Autodesk Inventor part; units mm, degrees
ref_plane "YZ Plane" through (0, 0, 0) normal (1, 0, 0) x (0, 1, 0)
ref_plane "XZ Plane" through (0, 0, 0) normal (0, 1, 0) x (-1, 0, 0)
ref_plane "XY Plane" through (0, 0, 0) normal (0, 0, 1) x (1, 0, 0)
sketch "Esboço1" plane through (0, 0, 0) normal (0, 1, 0) x (-1, 0, 0)
  line L0 (-40, 40) -> (40, 40)
  line L1 (40, 40) -> (40, -40)
  line L2 (40, -40) -> (-40, -40)
  line L3 (-40, -40) -> (-40, 40)
  line L4 (-40, 40) -> (40, -40) construction
  line L5 (40, 40) -> (-40, -40) construction
  point P0 (0, 0)
  dimension "d0" = 80
  dimension "d1" = 80
extrude "Extrusão1" add sketch "Esboço1" along normal blind 2.5
sketch "Esboço2" plane through (0, 2.5, 0) normal (0, 1, 0) x (1, 0, 0)
  circle A0 centre (33, -28) radius 1.5875
  line L0 (-40, -40) -> (40, -40)
  line L1 (40, -40) -> (40, 40)
  circle A1 centre (33, -0.06) radius 1.5875
  circle A2 centre (33, -28) radius 4.5
  circle A3 centre (33, -0.06) radius 4.5
  dimension "d4" = 3.175
  dimension "d5" = 12
  dimension "d6" = 7
  dimension "d7" = 3.175
  dimension "d8" = 27.94
  dimension "d9" = 9
  dimension "d10" = 9
extrude "Extrusão2" add sketch "Esboço2" along normal blind 3
sketch "Esboço3" plane through (0, 2.5, 0) normal (0, 1, 0) x (1, 0, 0)
  line L0 (-6.9727, -23.0834) -> (-13.0273, -23.0834)
  line L1 (-13.0273, -23.0834) -> (-13.0273, 3.9103)
  line L2 (-13.0273, 3.9103) -> (-6.9727, 3.9103)
  line L3 (-6.9727, 3.9103) -> (-6.9727, -23.0834)
  line L4 (-6.9727, -23.0834) -> (-13.0273, 3.9103) construction
  line L5 (-13.0273, -23.0834) -> (-6.9727, 3.9103) construction
  line L6 (40, -40) -> (40, 40)
  point P0 (0, 0)
  point P1 (-10, -9.5866)
  dimension "d13" = 50
extrude "Extrusão3" add sketch "Esboço3" along normal blind 3
sketch "Esboço4" plane through (0, 2.5, 0) normal (0, 1, 0) x (1, 0, 0)
  line L0 (13, 36) -> (-15, 36)
  line L1 (-15, 36) -> (-15, 22)
  line L2 (-15, 22) -> (13, 22)
  line L3 (13, 22) -> (13, 36)
  line L4 (35.54, 17.72) -> (-33.04, 17.72)
  line L5 (-33.04, 17.72) -> (-33.04, -35.62)
  line L6 (-33.04, -35.62) -> (35.54, -35.62)
  line L7 (35.54, -35.62) -> (35.54, 17.72)
  circle A0 centre (33, -28) radius 1.5875
  line L8 (15, 38) -> (-17, 38)
  line L9 (-17, 38) -> (-17, 20)
  line L10 (-17, 20) -> (15, 20)
  line L11 (15, 20) -> (15, 38)
  line L12 (40, 40) -> (-40, 40)
  line L13 (40, -40) -> (40, 40)
  point P0 (0, 0)
  dimension "d16" = 28
  dimension "d17" = 14
  dimension "d18" = 68.58
  dimension "d19" = 53.34
  dimension "d20" = 7.62
  dimension "d21" = 2.54
  dimension "d22" = 4
  dimension "d23" = 27
  dimension "d24" = 2
  dimension "d25" = 2
  dimension "d26" = 2
  dimension "d27" = 2
extrude "Extrusão4" add sketch "Esboço4" along normal blind 6 contours L11 L10 L9 L8
sketch "Esboço5" plane through (-17, 2.5, -20) normal (0, 0, 1) x (1, 0, 0)
  line L0 (0, 6) -> (32, 6)
  line L1 (3.1604, 6) -> (8.0765, 6)
  line L2 (8.0765, 6) -> (8.0765, 3)
  line L3 (8.0765, 3) -> (3.1604, 3)
  line L4 (3.1604, 3) -> (3.1604, 6)
  point P0 (17, -2.5)
  dimension "d32" = 3
extrude "Extrusão5" cut sketch "Esboço5" against normal blind 6
sketch "Esboço6" plane through (0, 2.5, 0) normal (0, 1, 0) x (1, 0, 0)
  line L0 (15, 20) -> (-17, 20)
  line L1 (-17, 20) -> (-27, 20)
  line L2 (-27, 20) -> (-27, 38)
  line L3 (-27, 38) -> (-17, 38)
  line L4 (-17, 38) -> (-17, 20)
  point P0 (0, 0)
  dimension "d33" = 10
extrude "Extrusão6" add sketch "Esboço6" along normal blind 6
fillet "Arredondamento1" radius 9 2 edges at (-27, 5.5, -20) (-27, 5.5, -38)
sketch "Esboço7" plane through (0, 8.5, 0) normal (0, 1, 0) x (1, 0, 0)
  circle A0 centre (-19.962, 29) radius 1.5
  point P0 (0, 0)
  dimension "d37" = 3
extrude "Extrusão7" cut sketch "Esboço7" against normal blind 6
sketch "Esboço8" plane through (0, 2.5, 0) normal (0, 1, 0) x (1, 0, 0)
  line L0 (-42.5, -42.5) -> (42.5, -42.5)
  line L1 (42.5, -42.5) -> (42.5, 42.5)
  line L2 (42.5, 42.5) -> (-42.5, 42.5)
  line L3 (-42.5, 42.5) -> (-42.5, -42.5)
  line L4 (40, 40) -> (-40, 40)
  line L5 (-40, 40) -> (-40, -40)
  line L6 (-40, -40) -> (40, -40)
  line L7 (40, -40) -> (40, 40)
  point P0 (0, 0)
  dimension "d40" = 2.5
  dimension "d41" = 2.5
  dimension "d42" = 2.5
  dimension "d43" = 2.5
extrude "Extrusão8" add sketch "Esboço8" along normal blind 25 and the other way blind 2.5
fillet "Arredondamento2" radius 2 4 edges at (-42.5, 13.75, 42.5) (-42.5, 13.75, -42.5) (42.5, 13.75, 42.5) (42.5, 13.75, -42.5)
sketch "Esboço10" plane through (-42.5, 0, -40.5) normal (-1, 0, 0) x (0, 0, 1)
  line L0 (76.52, 0) -> (23.18, 0)
  line L1 (81, 27.5) -> (81, 0)
  line L2 (0.5, 2.5) -> (80.5, 2.5)
  line L3 (32.58, 2.5) -> (47.58, 2.5)
  line L4 (47.58, 2.5) -> (47.58, 14.5)
  line L5 (47.58, 14.5) -> (32.58, 14.5)
  line L6 (32.58, 14.5) -> (32.58, 2.5)
  point P0 (40.5, 0)
  dimension "d51" = 15
  dimension "d52" = 12
extrude "Extrusão9" cut sketch "Esboço10" against normal blind 3
fillet "Arredondamento3" radius 2 2 edges at (-41.25, 14.5, 7.08) (-41.25, 14.5, -7.92)
sketch "Esboço11" plane through (0, 27.5, 0) normal (0, 1, 0) x (1, 0, 0)
  line L0 (40, -40) -> (40, 40)
  line L1 (40, 40) -> (34, 40)
  line L2 (34, 40) -> (34, 34)
  line L3 (34, 34) -> (40, 34)
  line L4 (40, 34) -> (40, 40)
  line L5 (-40, -7.08) -> (-40, -40)
  line L6 (-40, -40) -> (-34, -40)
  line L7 (-34, -40) -> (-34, -34)
  line L8 (-34, -34) -> (-40, -34)
  line L9 (-40, -34) -> (-40, -40)
  point P0 (0, 0)
  dimension "d57" = 6
  dimension "d58" = 6
  dimension "d59" = 6
  dimension "d60" = 6
extrude "Extrusão10" add sketch "Esboço11" against normal blind 25
fillet "Arredondamento4" radius 2 2 edges at (-34, 15, 34) (34, 15, -34)
sketch "Esboço12" plane through (0, 27.5, 0) normal (0, 1, 0) x (1, 0, 0)
  circle A0 centre (-38.25, -38.25) radius 1.5
  circle A1 centre (38.25, 38.25) radius 1.5
  line L0 (40.5, 42.5) -> (-40.5, 42.5)
  line L1 (42.5, -40.5) -> (42.5, 40.5)
  line L2 (-40.5, -42.5) -> (40.5, -42.5)
  line L3 (-42.5, 40.5) -> (-42.5, -40.5)
  point P0 (0, 0)
  dimension "d64" = 3
  dimension "d65" = 3
  dimension "d66" = 4.25
  dimension "d67" = 4.25
  dimension "d68" = 4.25
  dimension "d69" = 4.25
extrude "Extrusão11" cut sketch "Esboço12" against normal blind 10
sketch "Esboço13" plane through (40.5, 0, -42.5) normal (0, 0, -1) x (-1, 0, 0)
  circle A0 centre (73.7947, 8.7851) radius 2.5
  point P0 (40.5, 0)
  dimension "d72" = 5
extrude "Extrusão12" cut sketch "Esboço13" against normal blind 10
properties part number "caixa box"
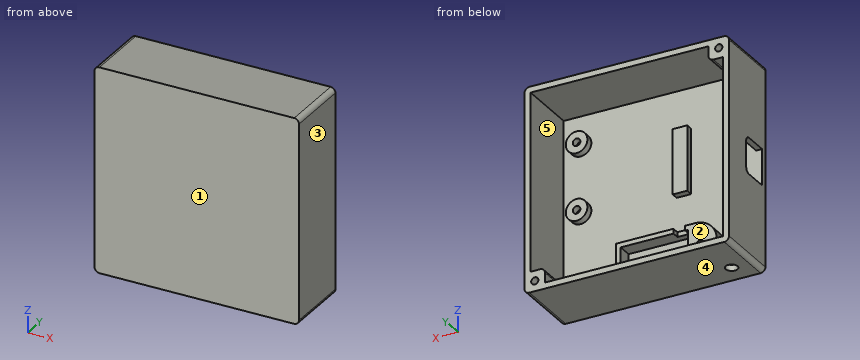
The model under review builds one solid part; all positions refer to its coordinate system, in mm. Face numbers are marked on the shaded views. A direction names the side the tool comes from. Coordinates: 2 decimals unless noted, no trailing zeros. Write each loop counter-clockwise with the first axis right and the second up, starting at its lowest first coordinate (ties: lowest second). Pieces come first, ordered by that corner, then holes. Notation, with made-up numbers: (22, 42.5) - (76, 42.5) arc R7 cw to (76, 53.5) - close; hole circle Ø1 at (66, -39.5). An arc over 180 degrees is marked (long way). Answer in a Markdown table with one row per item. Add a question column.
Q1. For the marked faces 1 and 2, list the 3-axis set-ups (+Z, -Z, +X, -X, +Y, -Y) from which the entire face can be reached by the end or side of a thin tool; tool diameter is ignored.
Q2. To check wall thickness, follow line 1 along X through (y, z) = (25, 38.25); line 2 along Z through (x, y) = (-38.25, 21); line 3 along X through (y, z) = (4.65, 0.06). State the ranges of each line that lie inside material, in increasing order. Write a range as from..to.
Q3. Clearance check with flat-ended pins moving along their axes: pin 1 (2 mm diameter, centred on x = -12, z = -21, fed in from +Y); pin 2 (8 mm diameter, centred on x = 33, z = -19.5, fed in from -Y); pin 3 (1 mm diameter, centred on x = -21.5, z = -22, fed in from +Y); pin 4 (0.8 mm diameter, centred on x = -41.5, y = 8.5, fed in from -Z). State where each tip first meets the part, or that it passes through.
Q4. Consider section B-B on y = 24.75. Give the boundary of the cut face in (x, z).
Q5. Draft analysis for pull direction X (two halves, no side actions). For the marked faces 3, 4 and 5, state which applies: +X half, -X half, draft (parallel to the pull), parting line (faces both ways), or undercut.
Q6. Consider section C-C on x = 4. Give the boundary of the cut face in (y, z).
Q7. Consider section A-A on z = 0.06. Give the boundary of the cut face in (x, y), then the cut area to 3 significant figures.
Q8. Consider section D-D on z = -10.5. Give the boundary of the cut face in (x, y), then the cut area to 4 significant figures.
Answers below:
| question | item | result |
|---|---|---|
| 1 | face 1 | +Z, -Z, +X, -X, -Y |
| 1 | face 2 | +Y |
| 2 | line 1 | -42.5..-39.75, -36.75..-34, 40..42.5 |
| 2 | line 2 | -42.5..-40, 34..36.75, 39.75..42.5 |
| 2 | line 3 | -13.03..-6.97, 28.5..31.41, 34.59..37.5, 40..42.5 |
| 3 | pin 1 | y = 5.5 |
| 3 | pin 2 | y = 0 |
| 3 | pin 3 | y = 8.5 |
| 3 | pin 4 | z = -42.41 |
| 4 | outline | (-42.5, -40.5) arc R2 ccw to (-40.5, -42.5) - (40.5, -42.5) arc R2 ccw to (42.5, -40.5) - (42.5, 40.5) arc R2 ccw to (40.5, 42.5) - (-40.5, 42.5) arc R2 ccw to (-42.5, 40.5) - close; hole (-40, -40) - (34, -40) - (34, -36) arc R2 cw to (36, -34) - (40, -34) - (40, 40) - (-34, 40) - (-34, 36) arc R2 cw to (-36, 34) - (-40, 34) - close; hole circle Ø3 at (-38.25, 38.25); hole circle Ø3 at (38.25, -38.25) |
| 5 | face 3 | +X half |
| 5 | face 4 | draft |
| 5 | face 5 | undercut |
| 6 | outline | (0, -42.5) - (27.5, -42.5) - (27.5, -40) - (2.5, -40) - (2.5, -38) - (8.5, -38) - (8.5, -36) - (2.5, -36) - (2.5, -22) - (8.5, -22) - (8.5, -20) - (2.5, -20) - (2.5, 40) - (27.5, 40) - (27.5, 42.5) - (0, 42.5) - close |
| 7 | outline | (-42.5, 0) - (42.5, 0) - (42.5, 27.5) - (40, 27.5) - (40, 2.5) - (37.5, 2.5) - (37.5, 5.5) - (34.59, 5.5) - (34.59, 2.5) - (31.41, 2.5) - (31.41, 5.5) - (28.5, 5.5) - (28.5, 2.5) - (-6.97, 2.5) - (-6.97, 5.5) - (-13.03, 5.5) - (-13.03, 2.5) - (-42.5, 2.5) - close; (-42.5, 14.5) - (-40, 14.5) - (-40, 27.5) - (-42.5, 27.5) - close |
| 7 | area | 343 mm² |
| 8 | outline | (-42.5, 0) - (42.5, 0) - (42.5, 27.5) - (40, 27.5) - (40, 2.5) - (-40, 2.5) - (-40, 27.5) - (-42.5, 27.5) - close |
| 8 | area | 337.5 mm² |
